Check sheet for the modelled part. Datum: model origin and axes. Units: mm. Give positions to 0.01 mm unless a question says otherwise; leave off trailing zeros. Order: outer loops, then holes, each group sorted by start corner. A loop starts at its lowest first (then second) coordinate and runs counter-clockwise, first axis right, second up.
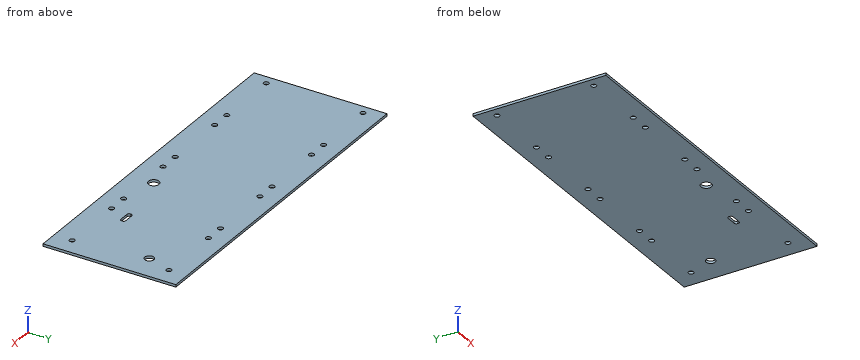
```python
from build123d import *

# Parameters (mm, degrees)
SKETCH_W   = 209.14
SKETCH_H   = 81.05
SKETCH_R   = 1.6
SKETCH_R_2 = 2.75
SKETCH_R_3 = 3.25
PAD_DEPTH  = 1.5


with BuildPart() as part:
    # Sketch → Pad (new body)
    with BuildSketch(Plane.XY):
        with Locations((104.57, 40.525)):
            Rectangle(SKETCH_W, SKETCH_H)
        with Locations((5.94, 70.05)):
            Circle(SKETCH_R, mode=Mode.SUBTRACT)
        with Locations((44.99, 70.05)):
            Circle(SKETCH_R, mode=Mode.SUBTRACT)
        with Locations((56.99, 70.05)):
            Circle(SKETCH_R, mode=Mode.SUBTRACT)
        with Locations((96.04, 70.05)):
            Circle(SKETCH_R, mode=Mode.SUBTRACT)
        with Locations((108.04, 70.05)):
            Circle(SKETCH_R, mode=Mode.SUBTRACT)
        with Locations((147.09, 70.05)):
            Circle(SKETCH_R, mode=Mode.SUBTRACT)
        with Locations((159.09, 70.05)):
            Circle(SKETCH_R, mode=Mode.SUBTRACT)
        with Locations((198.14, 70.05)):
            Circle(SKETCH_R, mode=Mode.SUBTRACT)
        with Locations((198.14, 11)):
            Circle(SKETCH_R, mode=Mode.SUBTRACT)
        with Locations((159.09, 11)):
            Circle(SKETCH_R, mode=Mode.SUBTRACT)
        with Locations((147.09, 11)):
            Circle(SKETCH_R, mode=Mode.SUBTRACT)
        with Locations((108.04, 11)):
            Circle(SKETCH_R, mode=Mode.SUBTRACT)
        with Locations((96.04, 11)):
            Circle(SKETCH_R, mode=Mode.SUBTRACT)
        with Locations((56.99, 11)):
            Circle(SKETCH_R, mode=Mode.SUBTRACT)
        with Locations((44.99, 11)):
            Circle(SKETCH_R, mode=Mode.SUBTRACT)
        with Locations((5.94, 11)):
            Circle(SKETCH_R, mode=Mode.SUBTRACT)
        with Locations((193.09, 55)):
            Circle(SKETCH_R_2, mode=Mode.SUBTRACT)
        with Locations((124.811676, 15.624069)):
            Circle(SKETCH_R_3, mode=Mode.SUBTRACT)
        with BuildLine():
            Line((160.09, 21), (166.09, 21))
            ThreePointArc((166.09, 21), (166.973883, 21.366117), (167.34, 22.25))
            Line((167.34, 22.75), (167.34, 22.25))
            ThreePointArc((167.34, 22.75), (166.973883, 23.633883), (166.09, 24))
            Line((160.09, 24), (166.09, 24))
            ThreePointArc((160.09, 24), (159.206117, 23.633883), (158.84, 22.75))
            Line((158.84, 22.75), (158.84, 22.250002))
            ThreePointArc((158.84, 22.250002), (159.206116, 21.366117), (160.09, 21))
        make_face(mode=Mode.SUBTRACT)
    extrude(amount=PAD_DEPTH)


solid = part.part
```
(1) Sectioned sample at A-A (y = 55). Enter the section's corners in (x, z).
(2) Thickness scan on L1, parallel to Y at x = 56.99, z = 0.7; L2, parallel to Y at x = 164, z = 1.2; L3, parallel to X at y = 14.5, z = 0.35. Record the ranges inside material, lowest first.
(3) Go/stop test with a flat-tipped pin: P1, Ø3.5, axis at x = 96.04, y = 70.05, coming from the +Z side. Record where the tip stops, or that it passes through.
Values follow:
1. outline: (0, 0) - (190.34, 0) - (190.34, 1.5) - (0, 1.5) - close; (195.84, 0) - (209.14, 0) - (209.14, 1.5) - (195.84, 1.5) - close
2. L1: y = 0 to 9.4, 12.6 to 68.45, 71.65 to 81.05
2. L2: y = 0 to 21, 24 to 81.05
2. L3: x = 0 to 121.76, 127.86 to 209.14
3. P1: stops at z = 1.5
